from build123d import *

# Parameters (mm, degrees)
SKETCH1_R           = 1.5
BOSS_EXTRUDE1_DEPTH = 3
SKETCH2_W           = 40
SKETCH2_H           = 30
BOSS_EXTRUDE2_DEPTH = 3
BOSS_EXTRUDE3_DEPTH = 40
CUT_EXTRUDE1_DEPTH  = 3
FILLET2_R           = 2.5


with BuildPart() as part:
    # Sketch1 → Boss-Extrude1 (new body)
    with BuildSketch(Plane(origin=(0, 0, 0), x_dir=(1, 0, 0), z_dir=(0, 1, 0))):
        with BuildLine():
            Line((40, 0), (40, 15))
            ThreePointArc((40, 15), (38.535533906, 18.535533906), (35, 20))
            Line((35, 20), (5, 20))
            ThreePointArc((5, 20), (1.464466094, 18.535533906), (0, 15))
            Line((0, 15), (0, 0))
            Line((0, 0), (40, 0))
        make_face()
        with Locations((5, 15)):
            Circle(SKETCH1_R, mode=Mode.SUBTRACT)
        with Locations((5, 5)):
            Circle(SKETCH1_R, mode=Mode.SUBTRACT)
        with Locations((35, 15)):
            Circle(SKETCH1_R, mode=Mode.SUBTRACT)
        with Locations((35, 5)):
            Circle(SKETCH1_R, mode=Mode.SUBTRACT)
    extrude(amount=BOSS_EXTRUDE1_DEPTH)

    # Sketch2 → Boss-Extrude2 (add)
    with BuildSketch(Plane.XY):
        with Locations((20, 15)):
            Rectangle(SKETCH2_W, SKETCH2_H)
    extrude(amount=BOSS_EXTRUDE2_DEPTH)

    # Sketch3 → Boss-Extrude3 (add)
    with BuildSketch(Plane(origin=(40, 0, 0), x_dir=(0, 0, -1), z_dir=(1, 0, 0))):
        Polygon((-3, 30), (-13.606601718, 40.606601718), (-11.485281374, 42.727922061), (2.656854249, 56.870057685), (4.424621202, 55.102290732), (-10.338834765, 40.338834765), (0, 30), align=None)
    extrude(amount=-BOSS_EXTRUDE3_DEPTH)

    # Sketch4 → Cut-Extrude1 (cut)
    with BuildSketch(Plane(origin=(0, 27.106601718, 27.106601718), x_dir=(1, 0, 0), z_dir=(0, 0.707106781, 0.707106781))):
        with BuildLine():
            Line((3, 42.091883092), (0, 42.091883092))
            Line((0, 42.091883092), (0, 39.091883092))
            ThreePointArc((0, 39.091883092), (0.878679656, 41.213203436), (3, 42.091883092))
        make_face()
        with BuildLine():
            Line((40, 42.091883092), (37, 42.091883092))
            ThreePointArc((37, 42.091883092), (39.121320344, 41.213203436), (40, 39.091883092))
            Line((40, 39.091883092), (40, 42.091883092))
        make_face()
    extrude(amount=-CUT_EXTRUDE1_DEPTH, mode=Mode.SUBTRACT)

    # Fillet2
    fillet2_edges = [part.edges().sort_by_distance(p)[0] for p in [
        (40, 3, -7.5),
        (38.535533906, 3, -18.535533906),
        (20, 3, -20),
        (1.464466094, 3, -18.535533906),
        (0, 16.5, 0),
        (40, 16.5, 0),
        (20, 30, 0),
        (0, 3, -7.5),
        (20, 3, 0),
    ]]
    fillet(fillet2_edges, radius=FILLET2_R)


solid = part.part
Could you check a few things on this model? Use its own coordinates, in mm. A direction names the side the tool comes from. Give positions to 0.01 mm unless a question says otherwise; leave off trailing zeros. Order: outer loops, then holes, each group sorted by start corner. A loop starts at its lowest first (then second) coordinate and runs counter-clockwise, first axis right, second up.
1. I need wall thicknesses on L1, parallel to X at y = 0.95, z = -5; L2, parallel to Z at x = 5, y = 1; L3, parallel to X at y = 1.35, z = -5. Which ranges of each line are inside material? Lowest first, please.
Answers below:
L1: x = 0.04 to 3.5, 6.5 to 33.5, 36.5 to 39.96
L2: z = -19.95 to -16.5, -13.5 to -6.5, -3.5 to 3
L3: x = 0.15 to 3.5, 6.5 to 33.5, 36.5 to 39.85
2. For pin 1 (1.5 mm diameter, centred on y = 23.5, z = 0, fed in from -X); pin 2 (10 mm diameter, centred on y = 44, z = -1, fed in from +X); pin 3 (3.5 mm diameter, centred on x = 5, z = -5, fed in from +Y); pin 4 (4 mm diameter, centred on x = 35, y = 15, fed in from -Z), each with a flat end and sliding along its axis, tell me the tip position at first contact or that it passes through.
Answers below:
pin 1: stops at x = 0.71
pin 2: passes through
pin 3: stops at y = 56.28
pin 4: stops at z = 0
3. Suppose I cut it at B-B (z = -12.5). Write out the boundary of the cut face in (x, y).
Answers below:
outline: (0, 0) - (40, 0) - (40, 0.5) arc R2.5 ccw to (37.5, 3) - (2.5, 3) arc R2.5 ccw to (0, 0.5) - close
4. Which directions (+Z, -Z, +X, -X, +Y, -Y) give clear straight access to the entire face, cutting with the end or side of a thin tool? Please do faces 1 (the cylindrical face through (39.287, 19.189, 0.752)), 2 (the cylindrical face through (6.386, 1.479, -4.425)), 3 (the flat face through (40, 36, 7)), 4 (the cylindrical face through (20.245, 3.713, -0.752)).
Answers below:
face 1: -Z, +X
face 2: -Y
face 3: +Z, -Z, +X, +Y, -Y
face 4: -Z, +X, -X
5. Suppose I cut it at A-A (x = 11). Write out the boundary of the cut face in (y, z).
Answers below:
outline: (0, -20) - (0.5, -20) arc R2.5 ccw to (3, -17.5) - (3, -2.5) arc R2.5 cw to (5.5, 0) - (28.96, 0) arc R2.5 ccw to (30.73, 0.73) - (40.34, 10.34) - (55.1, -4.42) - (56.87, -2.66) - (40.61, 13.61) - (30, 3) - (0, 3) - close
6. Thinking about a two-plate mould opening in Y: for faces 5 (the flat face through (20, 0, -9)), 6 (the flat face through (20, 36, 6)), 7 (the cylindrical face through (38.57, 0.25, -18.5)), which applies, +Y half, -Y half, draft (parallel to the pull), parting line (faces both ways), or undercut?
Answers below:
face 5: -Y half
face 6: undercut
face 7: draft
7. Suppose I cut it at C-C (y = 46). Write out the boundary of the cut face in (x, z).
Answers below:
outline: (0, 4.68) - (40, 4.68) - (40, 8.21) - (0, 8.21) - close
